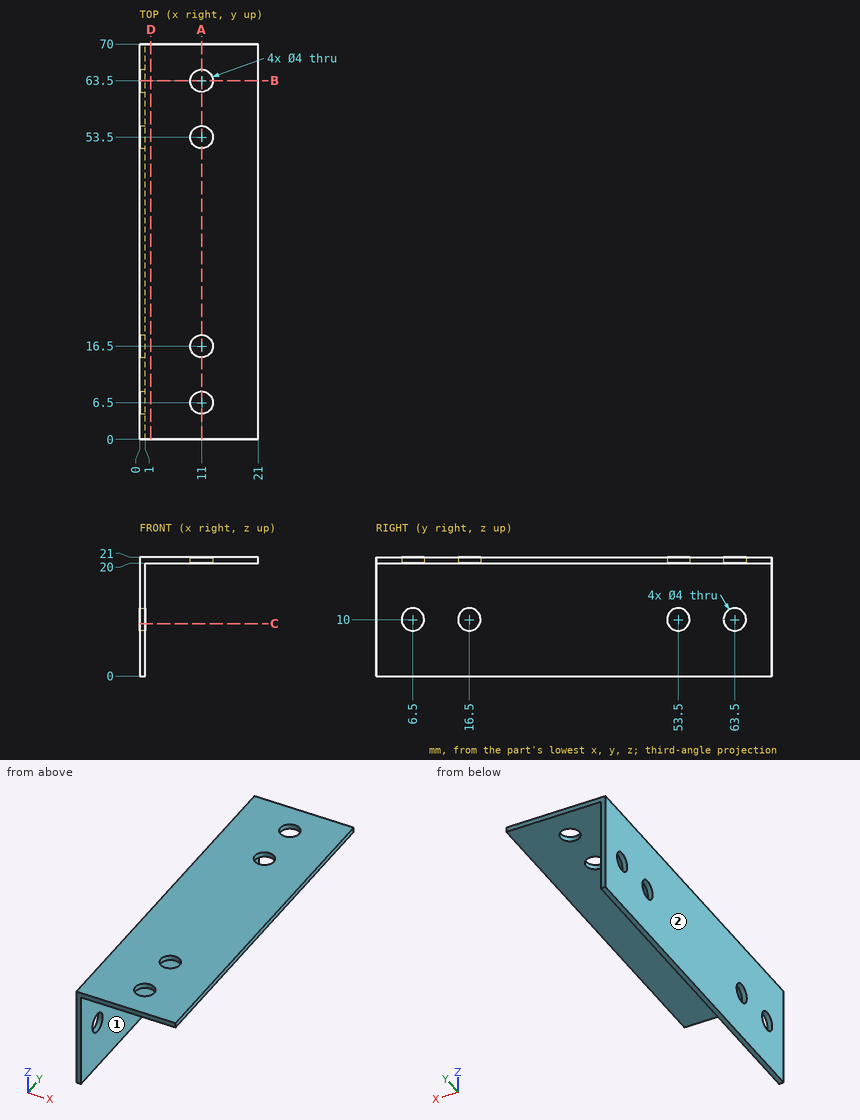
Input: dimensioned drawing with shaded views. Units: mm. Origin: part minimum x, y, z. A direction names the side the tool comes from. Give positions to 0.01 mm unless a question says otherwise; leave off trailing zeros. Loops run counter-clockwise (first coordinate to the right, second up) from the corner with the lowest first, then second, coordinate; pieces in that order, holes last. Notation, with made-up numbers: M 56,70.25 L 108,70.25 A22 ccw 108,80.25 Z; hole C -28,83 d9. An arc over 180 degrees is marked long. Put each result on its own line as item: value. Start each with the question number.
1) Cut plane A-A (x = 11). Output: boundary loops of the cut face in (y, z), then the cut area to 3 significant figures.
2) Cut plane D-D (x = 2). Output: boundary loops of the cut face in (y, z).
3) Access query for the marked faces 1 and 2. Directions: +Z, -Z, +X, -X, +Y, -Y. A direction counts if a zero-diameter tool reaches every point of the face in a straight line with its end or side. Return the directions, or none.
4) Cut plane B-B (y = 63.5). Output: boundary loops of the cut face in (x, z), then the cut area to 3 significant figures.
5) Contact query for flat-ended pins moving along their axis: pin 1 (5 mm diameter, centred on x = 11, y = 53.5, fed in from -Z); pin 2 (10 mm diameter, centred on y = 25, z = 13, fed in from +X). Output: stop coordinate, or through.
6) Cut plane C-C (z = 9.25). Output: boundary loops of the cut face in (x, y), then the cut area to 3 significant figures.
7) Ray query, line 1 along Y through (x, z) = (0.85, 10); line 2 along Z through (x, y) = (17.25, 34); line 3 along X through (y, z) = (52, 13.25). Return the intervals inside material, ascending.
Verdict:
1. outline: M 0,20 L 4.5,20 L 4.5,21 L 0,21 Z; M 8.5,20 L 14.5,20 L 14.5,21 L 8.5,21 Z; M 18.5,20 L 51.5,20 L 51.5,21 L 18.5,21 Z; M 55.5,20 L 61.5,20 L 61.5,21 L 55.5,21 Z; M 65.5,20 L 70,20 L 70,21 L 65.5,21 Z
1. area: 54.0 mm2
2. outline: M 0,20 L 70,20 L 70,21 L 0,21 Z
3. face 1: -Z, +X, +Y, -Y
3. face 2: +Z, -Z, -X, +Y, -Y
4. outline: M 0,0 L 1,0 L 1,8 L 0,8 Z; M 0,12 L 1,12 L 1,20 L 9,20 L 9,21 L 0,21 Z; M 13,20 L 21,20 L 21,21 L 13,21 Z
4. area: 33.0 mm2
5. pin 1: z = 20
5. pin 2: x = 1
6. outline: M 0,0 L 1,0 L 1,4.65 L 0,4.65 Z; M 0,8.35 L 1,8.35 L 1,14.65 L 0,14.65 Z; M 0,18.35 L 1,18.35 L 1,51.65 L 0,51.65 Z; M 0,55.35 L 1,55.35 L 1,61.65 L 0,61.65 Z; M 0,65.35 L 1,65.35 L 1,70 L 0,70 Z
6. area: 55.2 mm2
7. line 1: 0 to 4.5, 8.5 to 14.5, 18.5 to 51.5, 55.5 to 61.5, 65.5 to 70
7. line 2: 20 to 21
7. line 3: 0 to 1
